```python
from build123d import *

# Parameters (mm, degrees)
F1_DEPTH = 40
F2_R     = 7.5
F3_DEPTH = 5
F4_R     = 1


with BuildPart() as f1:
    # F0 (on Front) → F1 (new body)
    with BuildSketch(Plane.XZ):
        Polygon((-12.1263185228, 49.3127419949), (-32.1263185228, 49.3127419949), (-32.1263185228, -0.6872580051), (-12.1263185228, -0.6872580051), (-12.1263185228, 4.3127419949), (-27.1263185228, 4.3127419949), (-27.1263185228, 39.3127419949), (-12.1263185228, 39.3127419949), align=None)
    extrude(amount=F1_DEPTH)

    # F2 (on face) → F3 (cut)
    with BuildSketch(Plane.XY.offset(49.3127419949)):
        with Locations((-22.1263185228, -20)):
            Circle(F2_R)
    extrude(amount=-F3_DEPTH, mode=Mode.SUBTRACT)

    # F4
    f4_edges = [f1.edges().sort_by_distance(p)[0] for p in [
        (-22.126319, -40, 49.312742),
        (-12.126319, -20, 39.312742),
        (-12.126319, -20, 49.312742),
        (-12.126319, 0, 44.312742),
        (-12.126319, -40, 44.312742),
        (-22.126319, 0, 49.312742),
        (-32.126319, 0, 24.312742),
        (-22.126319, 0, -0.687258),
        (-12.126319, 0, 1.812742),
        (-19.626319, 0, 4.312742),
        (-27.126319, 0, 21.812742),
        (-19.626319, 0, 39.312742),
        (-12.126319, -20, 4.312742),
        (-27.126319, -20, 4.312742),
        (-19.626319, -40, 4.312742),
        (-32.126319, -20, -0.687258),
        (-12.126319, -20, -0.687258),
        (-22.126319, -40, -0.687258),
        (-12.126319, -40, 1.812742),
        (-27.126319, -40, 21.812742),
    ]]
    fillet(f4_edges, radius=F4_R)


solid = f1.part
```
Build history of the part. All positions in model axes, mm. A direction names the side the tool comes from. Give positions to 0.01 mm unless a question says otherwise; leave off trailing zeros. Loops run counter-clockwise (first coordinate to the right, second up) from the corner with the lowest first, then second, coordinate; pieces in that order, holes last.
1) Band-saw the part on A-A on x = -22. List the corners of the cut face in (y, z), then the cut area to 3 significant figures.
Values follow:
outline: (-40, 0.31) arc R1 ccw to (-39, -0.69) - (-1, -0.69) arc R1 ccw to (0, 0.31) - (0, 3.31) arc R1 ccw to (-1, 4.31) - (-39, 4.31) arc R1 ccw to (-40, 3.31) - close; (-40, 39.31) - (-1, 39.31) arc R1 ccw to (0, 40.31) - (0, 48.31) arc R1 ccw to (-1, 49.31) - (-12.5, 49.31) - (-12.5, 44.31) - (-27.5, 44.31) - (-27.5, 49.31) - (-39, 49.31) arc R1 ccw to (-40, 48.31) - close
area: 524 mm2
2) 3-axis set-ups, long thin cutter, end or side, ignore diameter. For faces 5 (the face through (-27.126, -20, 22)), 6 (the face through (-12.126, -20, 44)): which of +Z, -Z, +X, -X, +Y, -Y reach the whole face in a straight line?
Values follow:
face 5: +X, +Y, -Y
face 6: +Z, -Z, +X, +Y, -Y
3) Probe line 1 along Z through (x, y) = (-13.5, -34); line 2 along X through (y, z) = (-10, 39); line 3 along Z through (x, y) = (-19, -21). List the from-to ranges inside material, lowest first.
Values follow:
line 1: z = -0.69 to 4.31, 39.31 to 49.31
line 2: x = -32.13 to -27.13
line 3: z = -0.69 to 4.31, 39.31 to 44.31
4) Drop flat-ended pins along their axis: P1, Ø7.5, axis at x = -22, y = -19.5, coming from the +Z side; P2, Ø6, axis at x = -19, z = 34.5, coming from the +Y side. Give the stop position or say it passes through.
Values follow:
P1: stops at z = 44.31
P2: passes through
5) Band-saw the part on C-C on z = 34.5. List the corners of the cut face in (x, y), then the cut area to 3 significant figures.
Values follow:
outline: (-32.13, -40) - (-28.13, -40) arc R1 ccw to (-27.13, -39) - (-27.13, -1) arc R1 ccw to (-28.13, 0) - (-31.13, 0) arc R1 ccw to (-32.13, -1) - close
area: 199 mm2
6) Band-saw the part on D-D on x = -15.5. List the corners of the cut face in (y, z).
Values follow:
outline: (-40, 0.31) arc R1 ccw to (-39, -0.69) - (-1, -0.69) arc R1 ccw to (0, 0.31) - (0, 3.31) arc R1 ccw to (-1, 4.31) - (-39, 4.31) arc R1 ccw to (-40, 3.31) - close; (-40, 39.31) - (-1, 39.31) arc R1 ccw to (0, 40.31) - (0, 48.31) arc R1 ccw to (-1, 49.31) - (-16.49, 49.31) - (-16.49, 44.31) - (-23.51, 44.31) - (-23.51, 49.31) - (-39, 49.31) arc R1 ccw to (-40, 48.31) - close
7) Band-saw the part on B-B on y = -9.5. List the corners of the cut face in (x, z), then the cut area to 3 significant figures.
Values follow:
outline: (-32.13, 0.31) arc R1 ccw to (-31.13, -0.69) - (-13.13, -0.69) arc R1 ccw to (-12.13, 0.31) - (-12.13, 3.31) arc R1 ccw to (-13.13, 4.31) - (-26.13, 4.31) arc R1 cw to (-27.13, 5.31) - (-27.13, 39.31) - (-13.13, 39.31) arc R1 ccw to (-12.13, 40.31) - (-12.13, 48.31) arc R1 ccw to (-13.13, 49.31) - (-32.13, 49.31) - close
area: 474 mm2
8) Two-plate mould, pull along Y, no slides. Class faces 1 (the face through (-22, -20, 44.313)), 2 (the face through (-29, -24, 49.313)), 3 (the face through (-28.3, 0, 30)), 4 (the face through (-14.97, -17.75, 46.85)): released by +Y, released by -Y, zero draft, split by the parting line, or undercut.
Values follow:
face 1: undercut
face 2: zero draft
face 3: released by +Y
face 4: undercut
